Input: part model. Units: mm. Frame: model coordinates. Face numbers are marked on the shaded views. Give positions to 0.01 mm unless a question says otherwise; leave off trailing zeros. Order: outer loops, then holes, each group sorted by start corner. A loop starts at its lowest first (then second) coordinate and runs counter-clockwise, first axis right, second up. Notation, with made-up numbers: (-34, 56.25) - (24, 56.25) arc R15 cw to (24, 72.25) - close; hole circle Ø7 at (55, 5). An arc over 180 degrees is marked (long way). Answer in a Markdown table with one row per item. Add a question column.
1. Contact query for flat-ended pins moving along their axis: pin 1 (1.5 mm diameter, centred on x = -6, y = 4.5, fed in from -Z); pin 2 (10 mm diameter, centred on y = 14, z = -10, fed in from +X); pin 3 (2 mm diameter, centred on x = -15, z = 12.5, fed in from +Y); pin 4 (11 mm diameter, centred on x = 0, z = 0, fed in from +Y). Output: stop coordinate, or through.
2. Ray query, line 1 (X direction, y = 4.75, z = 0); line 2 (Z direction, x = -0.5, y = 6); line 3 (Z direction, x = 4, y = 14.25). Return the intervals inside material, ascending. Write a range as [from, to].
3. Section query D-D on z = 6. Return loops of the section in (x, y).
4. Section query A-A on z = 0. Return loops of the section in (x, y) (1 decimal), and give its area (3 significant figures).
5. Mould query, pull axis Z, two halves, no side actions, for the marked faces 1, 2, 3 and 4. Classes: released by +Z, released by -Z, zero draft, split by the parting line, or undercut.
6. Section query B-B on x = 0. Return loops of the section in (y, z) (1 decimal).
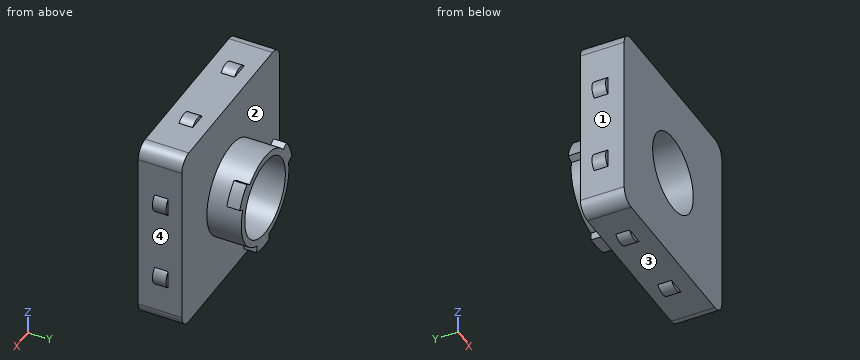
```python
from build123d import *

# Parameters (mm, degrees)
SKETCH1_W                = 44.29506
SKETCH1_H                = 44.29506
BOSS_EXTRUDE1_DEPTH      = 10.16
SKETCH2_R                = 10.795
SKETCH2_R_2              = 9.2075
BOSS_EXTRUDE2_DEPTH      = 8
BOSS_EXTRUDE3_START      = -3
BOSS_EXTRUDE3_DEPTH      = 3
CIRPATTERN1_COUNT        = 3
BOSS_EXTRUDE4_DEPTH      = 6.35
CUT_EXTRUDE1_DEPTH       = 3.175
LPATTERN1_COUNT          = 2
LPATTERN1_PITCH          = 19.05
FILLET1_R                = 3.175
CIRPATTERN2_COUNT        = 2
CIRPATTERN2_ANGLE        = 90
CIRPATTERN2_COPY_1_DEPTH = 6.35
CIRPATTERN2_COPY_2_DEPTH = 3.175
SKETCH13_R               = 9.2075
CUT_EXTRUDE2_DEPTH       = 35.245537666


with BuildPart() as part:
    # Sketch1 → Boss-Extrude1 (new body)
    with BuildSketch(Plane(origin=(0, 0, 0), x_dir=(1, 0, 0), z_dir=(0, 1, 0))):
        Rectangle(SKETCH1_W, SKETCH1_H)
    extrude(amount=BOSS_EXTRUDE1_DEPTH)

    # Sketch2 → Boss-Extrude2 (add)
    with BuildSketch(Plane(origin=(0, 10.16, 0), x_dir=(1, 0, 0), z_dir=(0, 1, 0))):
        with Locations(Location((0, 0, 0), (0, 0, 90))):
            Circle(SKETCH2_R)
        with Locations(Location((0, 0, 0), (0, 0, 270))):
            Circle(SKETCH2_R_2, mode=Mode.SUBTRACT)
    extrude(amount=BOSS_EXTRUDE2_DEPTH)

    # Sketch5 → Boss-Extrude3 (add)
    with BuildSketch(Plane(origin=(0, 18.16, 0), x_dir=(1, 0, 0), z_dir=(0, 1, 0)).offset(BOSS_EXTRUDE3_START)):
        with BuildLine():
            ThreePointArc((10.143998982, -3.692060354), (8.842746318, -6.19175763), (6.938853856, -8.269481977))
            Line((6.938853856, -8.269481977), (8.286221198, -9.212918747))
            ThreePointArc((8.286221198, -9.212918747), (10.150194049, -7.107242387), (11.491366324, -4.635497124))
            Line((11.491366324, -4.635497124), (10.143998982, -3.692060354))
        make_face()
    boss_extrude3 = extrude(amount=BOSS_EXTRUDE3_DEPTH)

    # CirPattern1: Boss-Extrude3 ×3 about axis
    cirpattern1_axis = Axis((0, 0, 0), (0, 1, 0))
    for i in range(1, CIRPATTERN1_COUNT):
        add(boss_extrude3.rotate(cirpattern1_axis, i * 360 / CIRPATTERN1_COUNT))

    # Sketch6 → Boss-Extrude4 (add)
    with BuildSketch(Plane(origin=(0, 10.16, 0), x_dir=(1, 0, 0), z_dir=(0, 1, 0))):
        with BuildLine():
            Line((-12.30653, 22.14753), (-7.98853, 22.14753))
            ThreePointArc((-7.98853, 22.14753), (-10.14753, 23.125), (-12.30653, 22.14753))
        make_face()
        with BuildLine():
            Line((-7.98853, -22.14753), (-12.30653, -22.14753))
            ThreePointArc((-12.30653, -22.14753), (-10.14753, -23.125), (-7.98853, -22.14753))
        make_face()
    boss_extrude4 = extrude(amount=-BOSS_EXTRUDE4_DEPTH)

    # Sketch7 → Cut-Extrude1 (cut)
    with BuildSketch(Plane(origin=(0, 10.16, 0), x_dir=(1, 0, 0), z_dir=(0, 1, 0))):
        with BuildLine():
            Line((-7.98853, 22.14753), (-12.30653, 22.14753))
            ThreePointArc((-12.30653, 22.14753), (-10.14753, 23.125), (-7.98853, 22.14753))
        make_face()
        with BuildLine():
            Line((-12.30653, -22.14753), (-7.98853, -22.14753))
            ThreePointArc((-7.98853, -22.14753), (-10.14753, -23.125), (-12.30653, -22.14753))
        make_face()
    cut_extrude1 = extrude(amount=-CUT_EXTRUDE1_DEPTH, mode=Mode.SUBTRACT)

    # LPattern1: Boss-Extrude4, Cut-Extrude1 ×2
    with Locations(*[(i * LPATTERN1_PITCH, 0, 0) for i in range(1, LPATTERN1_COUNT)]):
        add(boss_extrude4)
        add(cut_extrude1, mode=Mode.SUBTRACT)

    # Fillet1
    fillet1_edges = [part.edges().sort_by_distance(p)[0] for p in [
        (22.14753, 5.08, 22.14753),
        (-22.14753, 5.08, 22.14753),
        (-22.14753, 5.08, -22.14753),
        (22.14753, 5.08, -22.14753),
    ]]
    fillet(fillet1_edges, radius=FILLET1_R)

    # CirPattern2: Boss-Extrude4, Cut-Extrude1 ×2 about axis
    cirpattern2_axis = Axis((0, 0, 0), (0, -1, 0))
    add([boss_extrude4.rotate(cirpattern2_axis, i * CIRPATTERN2_ANGLE / (CIRPATTERN2_COUNT - 1)) for i in range(1, CIRPATTERN2_COUNT)])
    add([cut_extrude1.rotate(cirpattern2_axis, i * CIRPATTERN2_ANGLE / (CIRPATTERN2_COUNT - 1)) for i in range(1, CIRPATTERN2_COUNT)], mode=Mode.SUBTRACT)

    # CirPattern2 copy 1 sketch → CirPattern2 copy 1 (add)
    with BuildSketch(Plane(origin=(0, 10.16, 19.05), x_dir=(0, 0, 1), z_dir=(0, 1, 0))):
        with BuildLine():
            Line((-12.30653, 22.14753), (-7.98853, 22.14753))
            ThreePointArc((-7.98853, 22.14753), (-10.14753, 23.125), (-12.30653, 22.14753))
        make_face()
        with BuildLine():
            Line((-7.98853, -22.14753), (-12.30653, -22.14753))
            ThreePointArc((-12.30653, -22.14753), (-10.14753, -23.125), (-7.98853, -22.14753))
        make_face()
    extrude(amount=-CIRPATTERN2_COPY_1_DEPTH)

    # CirPattern2 copy 2 sketch → CirPattern2 copy 2 (cut)
    with BuildSketch(Plane(origin=(0, 10.16, 19.05), x_dir=(0, 0, 1), z_dir=(0, 1, 0))):
        with BuildLine():
            Line((-7.98853, 22.14753), (-12.30653, 22.14753))
            ThreePointArc((-12.30653, 22.14753), (-10.14753, 23.125), (-7.98853, 22.14753))
        make_face()
        with BuildLine():
            Line((-12.30653, -22.14753), (-7.98853, -22.14753))
            ThreePointArc((-7.98853, -22.14753), (-10.14753, -23.125), (-12.30653, -22.14753))
        make_face()
    extrude(amount=-CIRPATTERN2_COPY_2_DEPTH, mode=Mode.SUBTRACT)

    # Sketch13 → Cut-Extrude2 (cut, through all)
    with BuildSketch(Plane(origin=(0, 10.16, 0), x_dir=(1, 0, 0), z_dir=(0, 1, 0))):
        with Locations(Location((0, 0, 0), (0, 0, 270))):
            Circle(SKETCH13_R)
    extrude(amount=-CUT_EXTRUDE2_DEPTH, mode=Mode.SUBTRACT)


solid = part.part
```
Answer:
| question | item | result |
|---|---|---|
| 1 | pin 1 | stops at z = -22.15 |
| 1 | pin 2 | stops at x = 22.15 |
| 1 | pin 3 | stops at y = 10.16 |
| 1 | pin 4 | passes through |
| 2 | line 1 | x = [-22.15, -9.21], [9.21, 22.15] |
| 2 | line 2 | z = [-22.15, -9.19], [9.19, 22.15] |
| 2 | line 3 | z = [-10.03, -8.29], [8.29, 10.03] |
| 3 | outline | (-22.15, 0) - (-6.98, 0) - (-6.98, 18.16) - (-10.84, 18.16) - (-10.84, 15.16) - (-8.97, 15.16) - (-8.97, 10.16) - (-22.15, 10.16) - close; (6.98, 0) - (22.15, 0) - (22.15, 10.16) - (8.97, 10.16) - (8.97, 15.16) - (10.84, 15.16) - (10.84, 18.16) - (6.98, 18.16) - close |
| 4 | outline | (-22.1, 0) - (-9.2, 0) - (-9.2, 18.2) - (-10.8, 18.2) - (-10.8, 10.2) - (-22.1, 10.2) - close; (9.2, 0) - (22.1, 0) - (22.1, 10.2) - (10.8, 10.2) - (10.8, 18.2) - (9.2, 18.2) - close |
| 4 | area | 288 mm² |
| 5 | face 1 | undercut |
| 5 | face 2 | zero draft |
| 5 | face 3 | released by -Z |
| 5 | face 4 | undercut |
| 6 | outline | (0, -22.1) - (10.2, -22.1) - (10.2, -10.8) - (15.2, -10.8) - (15.2, -12.4) - (18.2, -12.4) - (18.2, -9.2) - (0, -9.2) - close; (0, 9.2) - (18.2, 9.2) - (18.2, 10.8) - (10.2, 10.8) - (10.2, 22.1) - (0, 22.1) - close |
